Job drawing, mm, ordinate dimensions from the low corner. One solid piece. A direction names the side the tool comes from. Give positions to 0.01 mm unless a question says otherwise; leave off trailing zeros. Loops run counter-clockwise (first coordinate to the right, second up) from the corner with the lowest first, then second, coordinate; pieces in that order, holes last.
Item 1: Probe probe 1 along Y at (x, z) = (80, 12.5); probe 2 along X at (y, z) = (6.75, 15.5); probe 3 along X at (y, z) = (5.5, 13). List the from-to ranges inside material, lowest first.
Item 2: Saw through at D-D on z = 14. Give the cut face in (x, y).
Item 3: Drop flat-ended pins along their axis: P1, Ø3, axis at x = 86.5, y = 10, coming from the +Z side; P2, Ø2, axis at x = 66.5, y = 13.5, coming from the +Z side; P3, Ø1, axis at y = 18, z = 32, coming from the -X side. Give the stop position or say it passes through.
Item 4: Which spindle directions (+Z, -Z, +X, -X, +Y, -Y) get a long thin tool onto all of the face, cutting with end or side? Do the marked faces 4, 5 and 6. Say none if no direction does.
Item 5: Saw through at B-B on z = 9. Give the cut face in (x, y), plus the area to 3 significant figures.
Item 6: Mould opens along Y. For the marked faces 1, 2 and 3 say: released by +Y, released by -Y, zero draft, split by the parting line, or undercut.
Item 7: Saw through at C-C on x = 6.5. Give the cut face in (y, z).
Item 8: Saw through at A-A on y = 10. Give the cut face in (x, z).
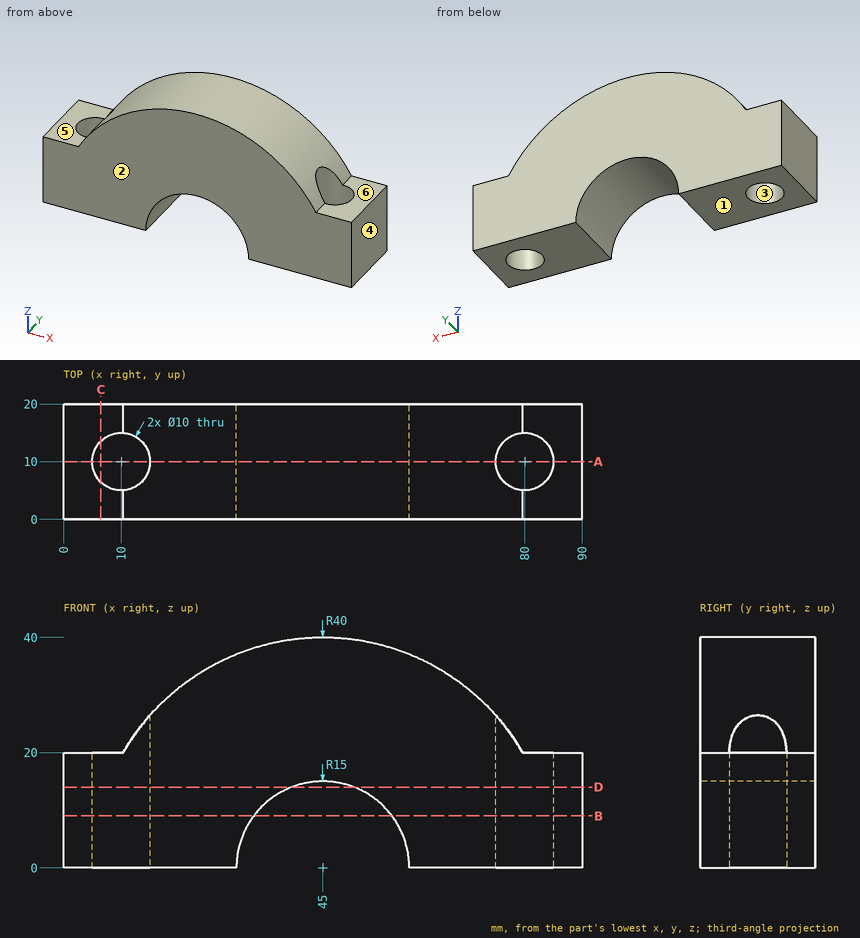
Results below:
1. probe 1: y = 0 to 5, 15 to 20
1. probe 2: x = 0 to 6.2, 13.8 to 76.2, 83.8 to 90
1. probe 3: x = 0 to 7.82, 12.18 to 37.52, 52.48 to 77.82, 82.18 to 90
2. outline: (0, 0) - (39.61, 0) - (39.61, 20) - (0, 20) - close; (50.39, 0) - (90, 0) - (90, 20) - (50.39, 20) - close; hole circle Ø10 at (10, 10); hole circle Ø10 at (80, 10)
3. P1: stops at z = 20
3. P2: stops at z = 34.35
3. P3: stops at x = 20.35
4. face 4: +Z, -Z, +X, +Y, -Y
4. face 5: +Z, -X, +Y, -Y
4. face 6: +Z, +X, +Y, -Y
5. outline: (0, 0) - (33, 0) - (33, 20) - (0, 20) - close; (57, 0) - (90, 0) - (90, 20) - (57, 20) - close; hole circle Ø10 at (10, 10); hole circle Ø10 at (80, 10)
5. area: 1,160 mm2
6. face 1: zero draft
6. face 2: released by -Y
6. face 3: undercut
7. outline: (0, 0) - (6.43, 0) - (6.43, 20) - (0, 20) - close; (13.57, 0) - (20, 0) - (20, 20) - (13.57, 20) - close
8. outline: (0, 0) - (5, 0) - (5, 20) - (0, 20) - close; (15, 0) - (30, 0) arc R15 cw to (60, 0) - (75, 0) - (75, 26.46) arc R40 ccw to (15, 26.46) - close; (85, 0) - (90, 0) - (90, 20) - (85, 20) - close
